Read the model definition and answer for the solid it produces. Units are mm, in the model's axes. Give positions to 0.01 mm unless a question says otherwise; leave off trailing zeros. Write each loop counter-clockwise with the first axis right and the second up, starting at its lowest first coordinate (ties: lowest second). Pieces come first, ordered by that corner, then holes. Notation, with made-up numbers: M 47.5,-4.75 L 100.5,-4.75 A24 cw 100.5,19.25 Z; hole C -11.5,-10 d1. An arc over 180 degrees is marked long. Use a Markdown table: item, result. Add a question column.
Item 1: A cutting plane is placed at C-C on z = 0.65. Count the separate pieces of the cut face and the enclosed holes in it, then the cut area to 3 significant figures.
Item 2: A cutting plane is placed at B-B on x = -20. Determine the outline of the cut face in (y, z), then the cut area to 3 significant figures.
Item 3: Consider probe 1 along Y at (x, z) = (1.5, 1); probe 2 along Y at (x, z) = (-75.08, 0.6); probe 3 along X at (y, z) = (-14, 0.9). Determine where each line is inside the solid, lowest interval first. Write a range as [from, to].
Item 4: Given P1, Ø0.9, axis at y = 4.5, z = 0.5, coming from the +X side; P2, Ø1.1, axis at x = 75.08, y = -10.84, coming from the +Z side; P3, Ø0.5, axis at x = -115, z = 1, coming from the +Y side, each flat-ended and moving along its own axis, determine where each tip first touches the part or whether it passes through.
Item 5: A cutting plane is placed at A-A on x = -92.5. Determine the outline of the cut face in (y, z), then the cut area to 3 significant figures.
from build123d import *

# Parameters (mm, degrees)
SKETCH1_R           = 0.9525
SKETCH1_W           = 2.54
SKETCH1_H           = 1.651
BOSS_EXTRUDE1_DEPTH = 1.7272
SKETCH3_W           = 1.7272
SKETCH3_H           = 2.032
BOSS_EXTRUDE2_DEPTH = 1.7272


with BuildPart() as part:
    # Sketch1 → Boss-Extrude1 (new body)
    with BuildSketch(Plane.XY):
        Polygon((-114.3, 13.37945), (-114.3, -13.37945), (-114.3, -15.91945), (114.3, -15.91945), (114.3, -13.37945), (114.3, 13.37945), (114.3, 15.91945), (-114.3, 15.91945), align=None)
        with Locations((-111.76, 10.83945)):
            Circle(SKETCH1_R, mode=Mode.SUBTRACT)
        with Locations(Location((-111.76, -10.83945, 0), (0, 0, 180))):
            Circle(SKETCH1_R, mode=Mode.SUBTRACT)
        with Locations((-75.08, 10.83945)):
            Circle(SKETCH1_R, mode=Mode.SUBTRACT)
        with Locations(Location((-75.08, -10.83945, 0), (0, 0, 180))):
            Circle(SKETCH1_R, mode=Mode.SUBTRACT)
        with Locations(Location((75.08, 10.83945, 0), (0, 0, 180))):
            Circle(SKETCH1_R, mode=Mode.SUBTRACT)
        with Locations(Location((111.76, 10.83945, 0), (0, 0, 180))):
            Circle(SKETCH1_R, mode=Mode.SUBTRACT)
        with Locations((111.76, -10.83945)):
            Circle(SKETCH1_R, mode=Mode.SUBTRACT)
        with Locations((75.08, -10.83945)):
            Circle(SKETCH1_R, mode=Mode.SUBTRACT)
        with BuildLine():
            Line((-107.95, -9.56945), (-80.16, -9.56945))
            ThreePointArc((-80.16, -9.56945), (-79.261974388, -9.197475612), (-78.89, -8.29945))
            Line((-78.89, -8.29945), (-78.89, 8.29945))
            ThreePointArc((-78.89, 8.29945), (-79.261974388, 9.197475612), (-80.16, 9.56945))
            Line((-80.16, 9.56945), (-107.95, 9.56945))
            ThreePointArc((-107.95, 9.56945), (-108.848025612, 9.197475612), (-109.22, 8.29945))
            Line((-109.22, 8.29945), (-109.22, -8.29945))
            ThreePointArc((-109.22, -8.29945), (-108.848025612, -9.197475612), (-107.95, -9.56945))
        make_face(mode=Mode.SUBTRACT)
        Polygon((-1.27, -8.93445), (-1.27, -2.088687016), (-53.255686673, -8.93445), align=None, mode=Mode.SUBTRACT)
        with BuildLine():
            Line((78.89, -8.29945), (78.89, 8.29945))
            ThreePointArc((78.89, 8.29945), (79.261974388, 9.197475612), (80.16, 9.56945))
            Line((80.16, 9.56945), (107.95, 9.56945))
            ThreePointArc((107.95, 9.56945), (108.848025612, 9.197475612), (109.22, 8.29945))
            Line((109.22, 8.29945), (109.22, -8.29945))
            ThreePointArc((109.22, -8.29945), (108.848025612, -9.197475612), (107.95, -9.56945))
            Line((107.95, -9.56945), (80.16, -9.56945))
            ThreePointArc((80.16, -9.56945), (79.261974388, -9.197475612), (78.89, -8.29945))
        make_face(mode=Mode.SUBTRACT)
        Polygon((-14.591172672, 0), (-72.54, 7.631022354), (-72.54, -7.631022354), align=None, mode=Mode.SUBTRACT)
        Polygon((-1.27, 8.93445), (-1.27, 2.088687016), (-53.255686673, 8.93445), align=None, mode=Mode.SUBTRACT)
        Polygon((1.27, -8.93445), (1.27, -2.088687016), (53.255686673, -8.93445), align=None, mode=Mode.SUBTRACT)
        Polygon((1.27, 8.93445), (1.27, 2.088687016), (53.255686673, 8.93445), align=None, mode=Mode.SUBTRACT)
        Polygon((14.591172672, 0), (72.54, -7.631022354), (72.54, 7.631022354), align=None, mode=Mode.SUBTRACT)
        with Locations((111.506, 14.45895)):
            Rectangle(SKETCH1_W, SKETCH1_H, mode=Mode.SUBTRACT)
        with Locations((111.506, -14.45895)):
            Rectangle(SKETCH1_W, SKETCH1_H, mode=Mode.SUBTRACT)
        with Locations((-111.506, 14.45895)):
            Rectangle(SKETCH1_W, SKETCH1_H, mode=Mode.SUBTRACT)
        with Locations((-111.506, -14.45895)):
            Rectangle(SKETCH1_W, SKETCH1_H, mode=Mode.SUBTRACT)
        with Locations((0, -14.45895)):
            Rectangle(SKETCH1_W, SKETCH1_H, mode=Mode.SUBTRACT)
        with Locations((0, 14.45895)):
            Rectangle(SKETCH1_W, SKETCH1_H, mode=Mode.SUBTRACT)
    extrude(amount=BOSS_EXTRUDE1_DEPTH)

    # Sketch3 → Boss-Extrude2 (add)
    with BuildSketch(Plane.XY):
        with Locations((-115.1636, 11.176)):
            Rectangle(SKETCH3_W, SKETCH3_H)
        with Locations((-115.1636, -11.176)):
            Rectangle(SKETCH3_W, SKETCH3_H)
        with Locations((115.1636, -11.176)):
            Rectangle(SKETCH3_W, SKETCH3_H)
        with Locations((115.1636, 11.176)):
            Rectangle(SKETCH3_W, SKETCH3_H)
    extrude(amount=BOSS_EXTRUDE2_DEPTH)


solid = part.part
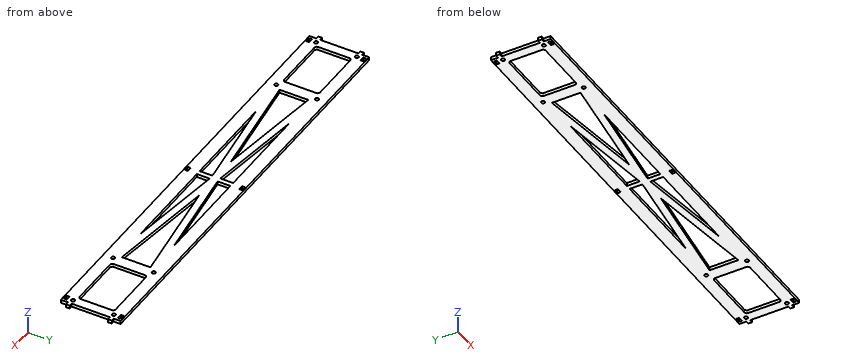
Filled in:
| question | item | result |
|---|---|---|
| 1 | separate pieces | 1 |
| 1 | enclosed holes | 22 |
| 1 | area | 4,490 mm² |
| 2 | outline | M -15.92,0 L -8.93,0 L -8.93,1.73 L -15.92,1.73 Z; M -4.56,0 L -0.71,0 L -0.71,1.73 L -4.56,1.73 Z; M 0.71,0 L 4.56,0 L 4.56,1.73 L 0.71,1.73 Z; M 8.93,0 L 15.92,0 L 15.92,1.73 L 8.93,1.73 Z |
| 2 | area | 37.4 mm² |
| 3 | probe 1 | [-15.92, -8.93], [-2.12, 2.12], [8.93, 15.92] |
| 3 | probe 2 | [-15.92, -11.79], [-9.89, 9.89], [11.79, 15.92] |
| 3 | probe 3 | [-114.3, -112.78], [-110.24, -1.27], [1.27, 110.24], [112.78, 114.3] |
| 4 | P1 | x = 114.3 |
| 4 | P2 | through |
| 4 | P3 | y = 12.19 |
| 5 | outline | M -15.92,0 L -9.57,0 L -9.57,1.73 L -15.92,1.73 Z; M 9.57,0 L 15.92,0 L 15.92,1.73 L 9.57,1.73 Z |
| 5 | area | 21.9 mm² |
